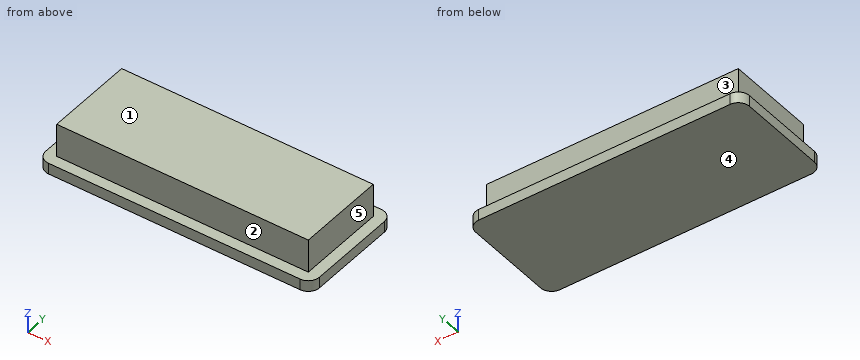
```python
from build123d import *

# Parameters (mm, degrees)
F0_W     = 115.316
F0_H     = 40.64
F1_DEPTH = 10.16
F2_W     = 125.476
F2_H     = 50.8
F2_W_2   = 115.316
F2_H_2   = 40.64
F3_DEPTH = 5.08
F4_R     = 5.08


with BuildPart() as f1:
    # F0 (on Top) → F1 (new body, symmetric)
    with BuildSketch(Plane.XY):
        with Locations((-0.381, 0.635)):
            Rectangle(F0_W, F0_H)
    extrude(amount=F1_DEPTH, both=True)

    # F2 (on face) → F3 (join)
    with BuildSketch(Plane(origin=(0, 0, -10.16), x_dir=(1, 0, 0), z_dir=(0, 0, -1))):
        with Locations((-0.381, -0.635)):
            Rectangle(F2_W, F2_H)
        with Locations((-0.381, -0.635)):
            Rectangle(F2_W_2, F2_H_2, mode=Mode.SUBTRACT)
    extrude(amount=-F3_DEPTH)

    # F4
    f4_edges = [f1.edges().sort_by_distance(p)[0] for p in [
        (-63.119, -24.765, -7.62),
        (62.357, -24.765, -7.62),
        (-63.119, 26.035, -7.62),
        (62.357, 26.035, -7.62),
    ]]
    fillet(f4_edges, radius=F4_R)


solid = f1.part
```
Verification items for the finished model (mm, model axes). Face numbers are marked on the shaded views. A direction names the side the tool comes from. Round coordinates to 2 decimals unless told otherwise and drop trailing zeros. Write each loop counter-clockwise with the first axis right and the second up, starting at its lowest first coordinate (ties: lowest second). Pieces come first, ordered by that corner, then holes. Notation, with made-up numbers: (16, 14.25) - (20, 14.25) arc R10 ccw to (20, 18.25) - close; hole circle Ø10 at (-12, 15.5). An arc over 180 degrees is marked (long way). Answer as a JSON object with one key per item and string values. Group by question number.
Q1. Section check A-A, the plane x = 38.5. Enter the section's corners in (y, z) (3 decimals), plus the area to 3 significant figures.
Q2. Section check C-C, the plane z = -1.25. Enter the section's corners in (x, y) (3 decimals).
Q3. Go/stop test with flat-tipped pins: pin 1 Ø10 at (x, z) = (16.5, 5) entering from +Y (3 decimals); pin 2 Ø7.5 at (x, z) = (5.5, -0.5) entering from -Y (3 decimals); pin 3 Ø7.5 at (y, z) = (-8, 1) entering from -X. Record where each tip stops, or that it passes through.
Q4. Section check B-B, the plane y = 11.5. Enter the section's corners in (x, z).
Q5. Thickness scan on line 1 (X direction, y = -19.5, z = -0.5); line 2 (Z direction, x = -27, y = 23.5); line 3 (Y direction, x = 24, z = -1) (3 decimals). Record the ranges inside material, lowest first.
Q6. Tool access check on the marked faces 1, 2, 3, 4 and 5. Record the directions out of +Z, -Z, +X, -X, +Y, -Y that give a thin tool (end or side, any length) a straight path to the whole face; none if there is none.
Found:
{
 "1": {"outline": "(-24.765, -10.16) - (26.035, -10.16) - (26.035, -5.08) - (20.955, -5.08) - (20.955, 10.16) - (-19.685, 10.16) - (-19.685, -5.08) - (-24.765, -5.08) - close", "area": "877 mm^2"},
 "2": {"outline": "(-58.039, -19.685) - (57.277, -19.685) - (57.277, 20.955) - (-58.039, 20.955) - close"},
 "3": {"pin 1": "stops at y = 20.955", "pin 2": "stops at y = -19.685", "pin 3": "stops at x = -58.04"},
 "4": {"outline": "(-63.12, -10.16) - (62.36, -10.16) - (62.36, -5.08) - (57.28, -5.08) - (57.28, 10.16) - (-58.04, 10.16) - (-58.04, -5.08) - (-63.12, -5.08) - close"},
 "5": {"line 1": "x = -58.04 to 57.28", "line 2": "z = -10.16 to -5.08", "line 3": "y = -19.685 to 20.955"},
 "6": {"face 1": "+Z, +X, -X, +Y, -Y", "face 2": "+Z, +X, -X, -Y", "face 3": "+Z, +X, -X, +Y", "face 4": "-Z, +X, -X, +Y, -Y", "face 5": "+Z, +X, +Y, -Y"}
}
